from build123d import *

# Parameters (mm, degrees)
F0_W     = 100
F0_H     = 75
F0_W_2   = 3
F0_H_2   = 10
F0_W_3   = 7
F0_H_3   = 4
F0_W_4   = 12
F0_H_4   = 15
F1_DEPTH = 2
F2_W     = 2
F2_H     = 40
F3_DEPTH = 25
F5_DEPTH = 100
F7_DEPTH = 100


with BuildPart() as f1:
    # F0 (on Front) → F1 (new body)
    with BuildSketch(Plane.XZ):
        with Locations((0, 5.5)):
            Rectangle(F0_W, F0_H)
        with Locations((-31.5, -17)):
            Rectangle(F0_W_2, F0_H_2, mode=Mode.SUBTRACT)
        with Locations((-11.5, -17)):
            Rectangle(F0_W_2, F0_H_2, mode=Mode.SUBTRACT)
        with Locations((11.5, -17)):
            Rectangle(F0_W_2, F0_H_2, mode=Mode.SUBTRACT)
        with Locations((31.5, -17)):
            Rectangle(F0_W_2, F0_H_2, mode=Mode.SUBTRACT)
        with Locations((0, -1)):
            Rectangle(F0_W_3, F0_H_3, mode=Mode.SUBTRACT)
        with Locations((-38, 15.5)):
            Rectangle(F0_W_4, F0_H_4, mode=Mode.SUBTRACT)
        with Locations((-16, 15.5)):
            Rectangle(F0_W_4, F0_H_4, mode=Mode.SUBTRACT)
        with Locations((16, 15.5)):
            Rectangle(F0_W_4, F0_H_4, mode=Mode.SUBTRACT)
        with Locations((38, 15.5)):
            Rectangle(F0_W_4, F0_H_4, mode=Mode.SUBTRACT)
        with Locations((0, 38)):
            Rectangle(F0_W_3, F0_H_3, mode=Mode.SUBTRACT)
    extrude(amount=F1_DEPTH)

    # F2 (on face) → F3 (join)
    with BuildSketch(Plane(origin=(0, 0, 0), x_dir=(-1, 0, 0), z_dir=(0, 1, 0))):
        with Locations((-49, 18)):
            Rectangle(F2_W, F2_H)
        with Locations((49, 18)):
            Rectangle(F2_W, F2_H)
    extrude(amount=-F3_DEPTH)

    # F4 (on face) → F5 (join)
    with BuildSketch(Plane(origin=(-50, 0, 0), x_dir=(0, -1, 0), z_dir=(-1, 0, 0))):
        Polygon((0, 43), (2, 43), (12, 63), (10, 63), align=None)
    extrude(amount=-F5_DEPTH)

    # F6 (on face) → F7 (cut)
    with BuildSketch(Plane.YZ.offset(50)):
        with BuildLine():
            Line((-7, 20.5), (-9, 20.5))
            ThreePointArc((-9, 20.5), (-14.5, 15), (-9, 9.5))
            Line((-9, 9.5), (-7, 9.5))
            ThreePointArc((-7, 9.5), (-1.5, 15), (-7, 20.5))
        make_face()
    extrude(amount=-F7_DEPTH, mode=Mode.SUBTRACT)


solid = f1.part
Geometry: final body of the model. Coordinates: model frame, mm. A direction names the side the tool comes from. Round coordinates to 2 decimals unless told otherwise and drop trailing zeros. Loops run counter-clockwise (first coordinate to the right, second up) from the corner with the lowest first, then second, coordinate; pieces in that order, holes last. Notation, with made-up numbers: M 75,0.5 L 88,0.5 A25 cw 88,19.5 Z; hole C 34.25,-28 d3. An arc over 180 degrees is marked long. Put each result on its own line as item: value. Start each with the question number.
(1) Draft query along Y for faces 1 (the face through (49, -14.5, 15.1)), 2 (the face through (1, 0, 6)), 3 (the face through (-26.9, -1.5, 15)), 4 (the face through (-49, -14.5, 15.1)). Return one class per face: +Y half, -Y half, draft (parallel to the pull), parting line (faces both ways), or undercut.
(2) Section query D-D (x = 5.5). Return loops of the section in (y, z), then the cut area to 3 significant figures.
(3) Section query C-C (y = -23). Return loops of the section in (x, z).
(4) Set-up query: faces 5 (the face through (48, -16, 18)), 6 (the face through (-1, -5, 53)), 7 (the face through (-47.6, -1.5, 14.9)). Return all of +Z, -Z, +X, -X, +Y, -Y with unobstructed straight access to the full face (end or side cutting, diameter ignored); none if empty.
(5) Section query B-B (z = 15). Return loops of the section in (x, y), then the cut area to 3 significant figures.
(6) Section query A-A (x = -17). Return loops of the section in (y, z).
(7) Material intervals for line 1 along X through (y, z) = (-10.75, -0.5); line 2 along Y through (x, z) = (-14, -23); line 3 along Y through (x, z) = (-15, 45), sorted ascending. Write a range as [from, to].
(8) Contact query for flat-ended pins moving along their axis: pin 1 Ø8 at (x, y) = (-4, -11.5) entering from -Z; pin 2 Ø2 at (x, y) = (-31, -1.5) entering from +Z; pin 3 Ø2 at (x, y) = (7, -13.5) entering from -Z; pin 4 Ø1.6 at (x, y) = (-49, -12.5) entering from +Z. Output: stop coordinate, or through.
Findings below:
1. face 1: undercut
1. face 2: +Y half
1. face 3: -Y half
1. face 4: undercut
2. outline: M -12,63 L -2,43 L -2,17.29 A5.5 cw -2,12.71 L -2,-32 L 0,-32 L 0,43 L -10,63 Z
2. area: 188 mm2
3. outline: M -50,-2 L -48,-2 L -48,38 L -50,38 Z; M 48,-2 L 50,-2 L 50,38 L 48,38 Z
4. face 5: -Z, -Y
4. face 6: +Z, +X, -X, +Y
4. face 7: +X, -X
5. outline: M -50,-25 L -48,-25 L -48,-14.5 L -50,-14.5 Z; M -50,-1.5 L -44,-1.5 L -44,0 L -50,0 Z; M -32,-1.5 L -22,-1.5 L -22,0 L -32,0 Z; M -10,-1.5 L 10,-1.5 L 10,0 L -10,0 Z; M 22,-1.5 L 32,-1.5 L 32,0 L 22,0 Z; M 44,-1.5 L 50,-1.5 L 50,0 L 44,0 Z; M 48,-25 L 50,-25 L 50,-14.5 L 48,-14.5 Z
5. area: 120 mm2
6. outline: M -12,63 L -2,43 L -2,23 L 0,23 L 0,43 L -10,63 Z; M -2,-32 L 0,-32 L 0,8 L -2,8 Z
7. line 1: x = [-50, -48], [48, 50]
7. line 2: y = [-2, 0]
7. line 3: y = [-3, -1]
8. pin 1: stops at z = 54
8. pin 2: stops at z = 48
8. pin 3: passes through
8. pin 4: stops at z = 63
